from build123d import *

# Parameters (mm, degrees)
SKETCH1_W           = 198
SKETCH1_H           = 173
BOSS_EXTRUDE1_DEPTH = 11
FILLET1_R           = 10
SKETCH2_W           = 12
SKETCH2_H           = 6.5
SKETCH2_W_2         = 16
SKETCH2_H_2         = 16.1
SKETCH2_H_3         = 6.2
SKETCH2_W_3         = 24
SKETCH2_W_4         = 31
CUT_EXTRUDE1_DEPTH  = 7


with BuildPart() as part:
    # Sketch1 → Boss-Extrude1 (new body)
    with BuildSketch(Plane(origin=(0, 0, 0), x_dir=(1, 0, 0), z_dir=(0, 1, 0))):
        Rectangle(SKETCH1_W, SKETCH1_H)
    extrude(amount=BOSS_EXTRUDE1_DEPTH)

    # Fillet1
    fillet1_edges = [part.edges().sort_by_distance(p)[0] for p in [
        (-99, 5.5, -86.5),
        (99, 5.5, -86.5),
        (99, 5.5, 86.5),
        (-99, 5.5, 86.5),
    ]]
    fillet(fillet1_edges, radius=FILLET1_R)

    # Sketch2 → Cut-Extrude1 (cut)
    with BuildSketch(Plane.XZ):
        with Locations((-65, 54.25)):
            Rectangle(SKETCH2_W, SKETCH2_H)
        with Locations((-36.2, 54.25)):
            Rectangle(SKETCH2_W, SKETCH2_H)
        with Locations((-63, 27.85)):
            Rectangle(SKETCH2_W_2, SKETCH2_H_2)
        with Locations((-63, 9)):
            Rectangle(SKETCH2_W_2, SKETCH2_H_3)
        with Locations((-35.2, 27.85)):
            Rectangle(SKETCH2_W_3, SKETCH2_H_2)
        with Locations((-35.2, 9)):
            Rectangle(SKETCH2_W_3, SKETCH2_H_3)
        with Locations((0, 27.85)):
            Rectangle(SKETCH2_W_4, SKETCH2_H_2)
    cut_extrude1 = extrude(amount=-CUT_EXTRUDE1_DEPTH, mode=Mode.SUBTRACT)

    # Mirror1: Cut-Extrude1 across plane
    add(cut_extrude1.mirror(Plane.ZY), mode=Mode.SUBTRACT)


solid = part.part
Source: CAD feature listing. Evaluate the final solid. Frame: model axes, mm. Round coordinates to 2 decimals unless told otherwise and drop trailing zeros. Order: outer loops, then holes, each group sorted by start corner. A loop starts at its lowest first (then second) coordinate and runs counter-clockwise, first axis right, second up. Notation, with made-up numbers: (57, -39.5) - (62, -39.5) arc R22 ccw to (62, -11.5) - close; hole circle Ø11 at (7, 85). An arc over 180 degrees is marked (long way). Use a Markdown table: item, result. Add a question column.
1. Section query A-A (z = 25.5). Return the cut outline in (x, y).
2. Section query C-C (y = 3). Give the number of separate pieces and of enclosed holes in the cut face, then the cut area to 3 significant figures.
3. Mould query, pull axis Z, two halves, no side actions, for faces 1 (the flat face through (99, 5, 1)), 2 (the cylindrical face through (96.15, 5.58, -83.49)), 3 (the flat face through (30.2, 3, 54)). Classes: +Z half, -Z half, draft (parallel to the pull), parting line (faces both ways), or undercut.
4. Line query: probe 1 along Z at (x, y) = (-65, 4.25); probe 2 along X at (y, z) = (5.25, 23); probe 3 along Z at (x, y) = (-42.5, 3). Output: solid intervals per line, ascending.
5. Section query B-B (x = -1). Return the cut outline in (y, z).
Derived:
| question | item | result |
|---|---|---|
| 1 | outline | (-99, 0) - (-71, 0) - (-71, 7) - (-55, 7) - (-55, 0) - (-47.2, 0) - (-47.2, 7) - (-23.2, 7) - (-23.2, 0) - (-15.5, 0) - (-15.5, 7) - (15.5, 7) - (15.5, 0) - (23.2, 0) - (23.2, 7) - (47.2, 7) - (47.2, 0) - (55, 0) - (55, 7) - (71, 7) - (71, 0) - (99, 0) - (99, 11) - (-99, 11) - close |
| 2 | separate pieces | 1 |
| 2 | enclosed holes | 13 |
| 2 | area | 31,600 mm2 |
| 3 | face 1 | draft |
| 3 | face 2 | -Z half |
| 3 | face 3 | undercut |
| 4 | probe 1 | -86.5 to 5.9, 12.1 to 19.8, 35.9 to 51, 57.5 to 86.5 |
| 4 | probe 2 | -99 to -71, -55 to -47.2, -23.2 to -15.5, 15.5 to 23.2, 47.2 to 55, 71 to 99 |
| 4 | probe 3 | -86.5 to 5.9, 12.1 to 19.8, 35.9 to 86.5 |
| 5 | outline | (0, -86.5) - (11, -86.5) - (11, 86.5) - (0, 86.5) - (0, 35.9) - (7, 35.9) - (7, 19.8) - (0, 19.8) - close |
